The listing builds one solid part. Answer for the finished solid, in the listing's coordinates (mm). A direction names the side the tool comes from. Give positions to 0.01 mm unless a question says otherwise; leave off trailing zeros. Loops run counter-clockwise (first coordinate to the right, second up) from the corner with the lowest first, then second, coordinate; pieces in that order, holes last.
Item 1: Section B-B, the plane x = 20 is taken. Give the number of separate pieces and of enclosed holes in the cut face, and give its area (3 significant figures).
Item 2: Each of these flat-tipped pins is pushed along its axis until it touches: pin 1 Ø1 at (x, z) = (3, 1.5) entering from -Y; pin 2 Ø1.5 at (x, z) = (14, 3.5) entering from +Y; pin 3 Ø1.5 at (y, z) = (14, 4) entering from +X. Where does it stop, or does it pass through?
Item 3: Section A-A, the plane y = 0 is taken. Give the vertices of the cut face in (x, z) (3 decimals).
Item 4: Consider line 1 along Y through (x, z) = (0, 3.6) (3 decimals); line 2 along Y through (x, z) = (0, 2.85) (3 decimals); line 3 along X through (y, z) = (2.5, 1.9). Determine where each line is inside the solid, lowest interval first.
Item 5: A tool of negligible diameter and unlimited length cuts with its end or side. For faces 1 (the face through (-10.9, -20.96, 2.5)), 2 (the face through (20.5, 8.59, 2.46)), from which of +Z, -Z, +X, -X, +Y, -Y can it reach the whole face along a straight path? Write none if from no direction.
from build123d import *

# Parameters (mm, degrees)
F0_R      = 27.305
F0_R_2    = 3.125
F1_DEPTH  = 5
F2_R      = 7.5
F2_R_2    = 3.125
F3_DEPTH  = 4
F4_R      = 6.096
F7_DEPTH  = 5.001
F10_R     = 0.662213
F11_DEPTH = 9.001
F12_W     = 13.650434
F12_H     = 4
F12_W_2   = 4
F12_H_2   = 13.650434
F13_DEPTH = 5
F15_DEPTH = 12.7
F16_W     = 10.29484
F16_H     = 1.244958
F17_DEPTH = 12.7
F18_R     = 8
F19_DEPTH = 12.7
F20_R     = 8
F21_DEPTH = 5


with BuildPart() as f1:
    # F0 (on Top) → F1 (new body)
    with BuildSketch(Plane.XY):
        Circle(F0_R)
        with BuildLine():
            Line((-10.097842, 16.405938), (-8.950036, 4.46059))
            ThreePointArc((-8.950036, 4.46059), (-10, 0), (-8.950036, -4.46059))
            Line((-8.950036, -4.46059), (-8.950036, -17.004333))
            ThreePointArc((-8.950036, -17.004333), (-9.992342, -18.76013), (-12.032858, -18.685849))
            ThreePointArc((-12.032858, -18.685849), (-22.211956, -0.761352), (-13.284091, 17.818068))
            ThreePointArc((-13.284091, 17.818068), (-11.278303, 18.043112), (-10.097842, 16.405938))
        make_face(mode=Mode.SUBTRACT)
        Circle(F0_R_2, mode=Mode.SUBTRACT)
        with BuildLine():
            Line((8.950036, 4.46059), (8.950036, 17.004333))
            ThreePointArc((8.950036, 17.004333), (9.992342, 18.76013), (12.032858, 18.685849))
            ThreePointArc((12.032858, 18.685849), (22.211956, 0.761352), (13.284091, -17.818068))
            ThreePointArc((13.284091, -17.818068), (11.278303, -18.043112), (10.097842, -16.405938))
            Line((10.097842, -16.405938), (8.950036, -4.46059))
            ThreePointArc((8.950036, -4.46059), (10, 0), (8.950036, 4.46059))
        make_face(mode=Mode.SUBTRACT)
    extrude(amount=F1_DEPTH)

    # F2 (on face) → F3 (join)
    with BuildSketch(Plane.XY.offset(5)):
        Circle(F2_R)
        Circle(F2_R_2, mode=Mode.SUBTRACT)
    extrude(amount=F3_DEPTH)

    # F4 (on Front) → F5 (revolve, cut)
    with BuildSketch(Plane.XZ):
        with Locations((-9.469913, 12.312098)):
            Circle(F4_R)
    revolve(axis=Axis((0, 0, 5.050069), (0, 0, -1)), mode=Mode.SUBTRACT)

    # F6 (on face) → F7 (cut, through all)
    with BuildSketch(Plane.XY.offset(5)):
        Polygon((0, 17.41166), (0, 11.362989), (5.234685, 11.362989), align=None)
        Polygon((-5.234685, 11.362989), (0, 11.362989), (0, 17.41166), align=None)
        Polygon((0, -11.362989), (-5.234685, -11.362989), (0, -17.41166), (5.234685, -11.362989), align=None)
    extrude(amount=-F7_DEPTH, mode=Mode.SUBTRACT)

    # F8 (on Front) → F9 (revolve, cut)
    with BuildSketch(Plane.XZ):
        Polygon((-25.495, 3.902024), (-25.495, 2.402024), (-23.495, 2.402024), align=None)
        Polygon((-23.495, 2.402024), (-25.495, 2.402024), (-25.495, 0.902024), align=None)
    revolve(axis=Axis((0, 0, 20.538263), (0, 0, -1)), mode=Mode.SUBTRACT)

    # F10 (on face) → F11 (cut, through all)
    with BuildSketch(Plane.XY):
        with Locations((0, 5.743192)):
            Circle(F10_R)
        with Locations((-4.06105, 4.06105)):
            Circle(F10_R)
        with Locations((-5.743192, 0)):
            Circle(F10_R)
        with Locations((-4.06105, -4.06105)):
            Circle(F10_R)
        with Locations((0, -5.743192)):
            Circle(F10_R)
        with Locations((4.06105, -4.06105)):
            Circle(F10_R)
        with Locations((5.743192, 0)):
            Circle(F10_R)
        with Locations((4.06105, 4.06105)):
            Circle(F10_R)
    extrude(amount=F11_DEPTH, mode=Mode.SUBTRACT)

    # F12 (on Top) → F13 (join)
    with BuildSketch(Plane.XY):
        with Locations((-15.625295, 0)):
            Rectangle(F12_W, F12_H)
        Polygon((-14.460696, -17.289123), (-4.808381, -7.636809), (-7.636809, -4.808381), (-17.289123, -14.460696), align=None)
        with Locations((0, -15.625295)):
            Rectangle(F12_W_2, F12_H_2)
        Polygon((17.289123, -14.460696), (7.636809, -4.808381), (4.808381, -7.636809), (14.460696, -17.289123), align=None)
        with Locations((15.625295, 0)):
            Rectangle(F12_W, F12_H)
        Polygon((14.460696, 17.289123), (4.808381, 7.636809), (7.636809, 4.808381), (17.289123, 14.460696), align=None)
        with Locations((0, 15.625295)):
            Rectangle(F12_W_2, F12_H_2)
        Polygon((-17.289123, 14.460696), (-7.636809, 4.808381), (-4.808381, 7.636809), (-14.460696, 17.289123), align=None)
    extrude(amount=F13_DEPTH)

    # F14 (on Top) → F15 (cut, symmetric)
    with BuildSketch(Plane.XY):
        with BuildLine():
            add(Edge.make_bspline(
                [(4.797351, 18.771529), (4.797351, 20.801119), (-2.398675, 19.786324), (-9.594701, 18.771529), (-2.398675, 17.756734), (4.797351, 16.74194), (4.797351, 18.771529)],
                knots=[0, 0, 0, 2.094395, 2.094395, 4.18879, 4.18879, 6.283185, 6.283185, 6.283185], degree=2, weights=[1, 0.5, 1, 0.5, 1, 0.5, 1]))
        make_face()
        with BuildLine():
            add(Edge.make_bspline(
                [(-4.797351, -18.771529), (-4.797351, -20.801119), (2.398675, -19.786324), (9.594701, -18.771529), (2.398675, -17.756734), (-4.797351, -16.74194), (-4.797351, -18.771529)],
                knots=[0, 0, 0, 2.094395, 2.094395, 4.18879, 4.18879, 6.283185, 6.283185, 6.283185], degree=2, weights=[1, 0.5, 1, 0.5, 1, 0.5, 1]))
        make_face()
    extrude(amount=F15_DEPTH, both=True, mode=Mode.SUBTRACT)

    # F16 (on Top) → F17 (cut, symmetric)
    with BuildSketch(Plane.XY):
        with Locations((0, 9.133866)):
            Rectangle(F16_W, F16_H)
        with Locations((0, -9.133866)):
            Rectangle(F16_W, F16_H)
    extrude(amount=F17_DEPTH, both=True, mode=Mode.SUBTRACT)

    # F18 (on face) → F19 (cut, symmetric)
    with BuildSketch(Plane.XY.offset(5)):
        Circle(F18_R)
    extrude(amount=F19_DEPTH, both=True, mode=Mode.SUBTRACT)

    # F20 (on face) → F21 (join)
    with BuildSketch(Plane.XY.offset(5)):
        with BuildLine():
            ThreePointArc((-2.194021, -9.756345), (0, -10), (2.194021, -9.756345))
            Line((2.194021, -9.756345), (-2.194021, -9.756345))
        make_face()
        with BuildLine():
            Line((5.14742, 8.511387), (5.14742, 8.573451))
            ThreePointArc((5.14742, 8.573451), (3.718064, 9.283103), (2.194021, 9.756345))
            Line((2.194021, 9.756345), (-2.194021, 9.756345))
            ThreePointArc((-2.194021, 9.756345), (-3.718064, 9.283103), (-5.14742, 8.573451))
            Line((-5.14742, 8.573451), (-5.14742, 8.511387))
            Line((-5.14742, 8.511387), (5.14742, 8.511387))
        make_face()
        with BuildLine():
            ThreePointArc((9.797959, -2), (9.949362, -1.00509), (10, 0))
            ThreePointArc((10, 0), (9.949362, 1.00509), (9.797959, 2))
            ThreePointArc((9.797959, 2), (9.454388, 3.257998), (8.950036, 4.46059))
            ThreePointArc((8.950036, 4.46059), (7.342579, 6.788706), (5.14742, 8.573451))
            Line((5.14742, 8.573451), (5.14742, 8.511387))
            Line((5.14742, 8.511387), (-5.14742, 8.511387))
            Line((-5.14742, 8.511387), (-5.14742, 8.573451))
            ThreePointArc((-5.14742, 8.573451), (-7.342579, 6.788706), (-8.950036, 4.46059))
            ThreePointArc((-8.950036, 4.46059), (-9.454388, 3.257998), (-9.797959, 2))
            ThreePointArc((-9.797959, 2), (-10, 0), (-9.797959, -2))
            ThreePointArc((-9.797959, -2), (-9.454388, -3.257998), (-8.950036, -4.46059))
            ThreePointArc((-8.950036, -4.46059), (-7.342579, -6.788706), (-5.14742, -8.573451))
            Line((-5.14742, -8.573451), (-5.14742, -8.511387))
            Line((-5.14742, -8.511387), (5.14742, -8.511387))
            Line((5.14742, -8.511387), (5.14742, -8.573451))
            ThreePointArc((5.14742, -8.573451), (7.342579, -6.788706), (8.950036, -4.46059))
            ThreePointArc((8.950036, -4.46059), (9.454388, -3.257998), (9.797959, -2))
        make_face()
        Circle(F20_R, mode=Mode.SUBTRACT)
        with BuildLine():
            ThreePointArc((2.194021, -9.756345), (3.718064, -9.283103), (5.14742, -8.573451))
            Line((5.14742, -8.573451), (5.14742, -8.511387))
            Line((5.14742, -8.511387), (-5.14742, -8.511387))
            Line((-5.14742, -8.511387), (-5.14742, -8.573451))
            ThreePointArc((-5.14742, -8.573451), (-3.718064, -9.283103), (-2.194021, -9.756345))
            Line((-2.194021, -9.756345), (2.194021, -9.756345))
        make_face()
        with BuildLine():
            Line((-2.194021, 9.756345), (2.194021, 9.756345))
            ThreePointArc((2.194021, 9.756345), (0, 10), (-2.194021, 9.756345))
        make_face()
    extrude(amount=-F21_DEPTH)


solid = f1.part
Worked answers:
1. separate pieces: 3
1. enclosed holes: 2
1. area: 98.8 mm2
2. pin 1: stops at y = -27.19
2. pin 2: stops at y = 23.87
2. pin 3: stops at x = 23.87
3. outline: (-27.305, 0) - (-8, 0) - (-8, 5) - (-27.305, 5) - close; (8, 0) - (27.305, 0) - (27.305, 5) - (8, 5) - close; hole (-25.495, 0.902) - (-23.495, 2.402) - (-25.495, 3.902) - close; hole (23.495, 2.402) - (25.495, 0.902) - (25.495, 3.902) - close
4. line 1: y = -27.305 to -25.495, -25.092 to -19.943, -17.6 to -8, 8 to 17.6, 19.943 to 25.092, 25.495 to 27.305
4. line 2: y = -27.305 to -25.495, -24.092 to -19.943, -17.6 to -8, 8 to 17.6, 19.943 to 24.092, 25.495 to 27.305
4. line 3: x = -27.19 to -25.37, -24.03 to -22.08, -9.68 to -7.6, 7.6 to 9.68, 22.08 to 24.03, 25.37 to 27.19
5. face 1: none
5. face 2: +Z, -Z
